Geometry: final body of the model. Coordinates: model frame, mm. A direction names the side the tool comes from. Give positions to 0.01 mm unless a question says otherwise; leave off trailing zeros. Write each loop counter-clockwise with the first axis right and the second up, starting at its lowest first coordinate (ties: lowest second). Pieces come first, ordered by that corner, then holes.
Q1. Cut plane D-D on x = 37. Return the cut outline in (y, z), plus the area to 3 significant figures.
Q2. Cut plane B-B on y = 41.5. Return the cut outline in (x, z).
Q3. Reachability of faces 1 (the face through (61.743, 36, 3)), 2 (the face through (-79.29, 59, 5.42)) from +Z, -Z, +X, -X, +Y, -Y: full face, straight path, thin tool, end or side. Return the list, or none.
Q4. Pin query (flat end, axial travel): pin 1 (2 mm diameter, centred on x = -70.5, y = 29, fed in from +Z). Return the tip coordinate at first contact, or that it passes through.
Q5. Cut plane A-A on z = 4.75. Count the separate pieces of the cut face and the enclosed holes in it, plus the area to 3 significant figures.
Q6. Cut plane C-C on x = -43. Return the cut outline in (y, z), plus the area to 3 significant figures.
Q7. Line query: L1, parallel to Y at x = -48, z = 8; L2, parallel to Y at x = -55, z = 5.5; L3, parallel to X at y = 15.5, z = 0.75. Output: solid intervals per line, ascending.
Q8. Draft query along Y for faces 3 (the face through (47, 48, 0)), 4 (the face through (-92.257, 36, 3)), 5 (the face through (-65, 26, 0)). Return one class per face: pulls with the +Y half, pulls with the -Y half, needs draft (parallel to the pull), parting line crosses it, or undercut.
```python
from build123d import *

# Parameters (mm, degrees)
F0_W     = 154
F0_H     = 50.650635
F0_R     = 11.75
F1_DEPTH = 4
F2_DEPTH = 11


with BuildPart() as f1:
    # F0 (on Top) → F1 (new body)
    with BuildSketch(Plane.XY):
        with Locations((-15.256856, 36.523289)):
            Rectangle(F0_W, F0_H)
        with Locations((-65.256856, 25.697972)):
            Circle(F0_R, mode=Mode.SUBTRACT)
        with Locations((-40.256856, 25.697972)):
            Circle(F0_R, mode=Mode.SUBTRACT)
        with Locations((-15.256856, 25.697972)):
            Circle(F0_R, mode=Mode.SUBTRACT)
        with Locations((9.743144, 25.697972)):
            Circle(F0_R, mode=Mode.SUBTRACT)
        with Locations((34.743144, 25.697972)):
            Circle(F0_R, mode=Mode.SUBTRACT)
        with Locations((-77.756856, 47.348607)):
            Circle(F0_R, mode=Mode.SUBTRACT)
        with Locations((-52.756856, 47.348607)):
            Circle(F0_R, mode=Mode.SUBTRACT)
        with Locations((-27.756856, 47.348607)):
            Circle(F0_R, mode=Mode.SUBTRACT)
        with Locations((-2.756856, 47.348607)):
            Circle(F0_R, mode=Mode.SUBTRACT)
        with Locations((22.243144, 47.348607)):
            Circle(F0_R, mode=Mode.SUBTRACT)
        with Locations((47.243144, 47.348607)):
            Circle(F0_R, mode=Mode.SUBTRACT)
        with Locations((-77.756856, 47.348607)):
            Circle(F0_R)
        with Locations((-65.256856, 25.697972)):
            Circle(F0_R)
        with Locations((-52.756856, 47.348607)):
            Circle(F0_R)
        with Locations((-40.256856, 25.697972)):
            Circle(F0_R)
        with Locations((-27.756856, 47.348607)):
            Circle(F0_R)
        with Locations((-2.756856, 47.348607)):
            Circle(F0_R)
        with Locations((-15.256856, 25.697972)):
            Circle(F0_R)
        with Locations((9.743144, 25.697972)):
            Circle(F0_R)
        with Locations((47.243144, 47.348607)):
            Circle(F0_R)
        with Locations((34.743144, 25.697972)):
            Circle(F0_R)
        with Locations((22.243144, 47.348607)):
            Circle(F0_R)
    extrude(amount=-F1_DEPTH)

    # F0 (on Top) → F2 (join)
    with BuildSketch(Plane.XY):
        with Locations((-15.256856, 36.523289)):
            Rectangle(F0_W, F0_H)
        with Locations((-65.256856, 25.697972)):
            Circle(F0_R, mode=Mode.SUBTRACT)
        with Locations((-40.256856, 25.697972)):
            Circle(F0_R, mode=Mode.SUBTRACT)
        with Locations((-15.256856, 25.697972)):
            Circle(F0_R, mode=Mode.SUBTRACT)
        with Locations((9.743144, 25.697972)):
            Circle(F0_R, mode=Mode.SUBTRACT)
        with Locations((34.743144, 25.697972)):
            Circle(F0_R, mode=Mode.SUBTRACT)
        with Locations((-77.756856, 47.348607)):
            Circle(F0_R, mode=Mode.SUBTRACT)
        with Locations((-52.756856, 47.348607)):
            Circle(F0_R, mode=Mode.SUBTRACT)
        with Locations((-27.756856, 47.348607)):
            Circle(F0_R, mode=Mode.SUBTRACT)
        with Locations((-2.756856, 47.348607)):
            Circle(F0_R, mode=Mode.SUBTRACT)
        with Locations((22.243144, 47.348607)):
            Circle(F0_R, mode=Mode.SUBTRACT)
        with Locations((47.243144, 47.348607)):
            Circle(F0_R, mode=Mode.SUBTRACT)
    extrude(amount=F2_DEPTH)


solid = f1.part
```
Data:
1. outline: (11.2, -4) - (61.85, -4) - (61.85, 11) - (53.11, 11) - (53.11, 0) - (41.59, 0) - (41.59, 11) - (37.23, 11) - (37.23, 0) - (14.17, 0) - (14.17, 11) - (11.2, 11) - close
1. area: 379 mm2
2. outline: (-92.26, -4) - (61.74, -4) - (61.74, 11) - (57.43, 11) - (57.43, 0) - (37.05, 0) - (37.05, 11) - (32.43, 11) - (32.43, 0) - (12.05, 0) - (12.05, 11) - (7.43, 11) - (7.43, 0) - (-12.95, 0) - (-12.95, 11) - (-17.57, 11) - (-17.57, 0) - (-37.95, 0) - (-37.95, 11) - (-42.57, 11) - (-42.57, 0) - (-62.95, 0) - (-62.95, 11) - (-67.57, 11) - (-67.57, 0) - (-87.95, 0) - (-87.95, 11) - (-92.26, 11) - close
3. face 1: +Z, -Z, +X, +Y, -Y
3. face 2: +Z
4. pin 1: stops at z = 0
5. separate pieces: 1
5. enclosed holes: 11
5. area: 3,030 mm2
6. outline: (11.2, -4) - (61.85, -4) - (61.85, 11) - (53.9, 11) - (53.9, 0) - (40.8, 0) - (40.8, 11) - (37.12, 11) - (37.12, 0) - (14.27, 0) - (14.27, 11) - (11.2, 11) - close
6. area: 364 mm2
7. L1: y = 11.2 to 16.86, 34.54 to 36.6, 58.09 to 61.85
7. L2: y = 11.2 to 19.97, 31.43 to 35.81, 58.88 to 61.85
7. L3: x = -92.26 to -71.09, -59.42 to -46.09, -34.42 to -21.09, -9.42 to 3.91, 15.58 to 28.91, 40.58 to 61.74
8. face 3: undercut
8. face 4: needs draft
8. face 5: undercut
